```python
from build123d import *

# Parameters (mm, degrees)
SKETCH1_W                      = 600
SKETCH1_H                      = 600
BOSS_EXTRUDE1_DEPTH            = 60
BOSS_EXTRUDE2_START            = 100
SKETCH2_R                      = 20
BOSS_EXTRUDE2_DEPTH            = 100
BOSS_EXTRUDE3_START            = -200
SKETCH2_2_R                    = 20
BOSS_EXTRUDE3_DEPTH            = 100
CUT_EXTRUDE1_REACH             = 677.574
SKETCH2_3_R                    = 20
CUT_EXTRUDE1_DIRECTION_2_REACH = 677.574
FILLET1_R                      = 50


with BuildPart() as part:
    # Sketch1 → Boss-Extrude1 (new body)
    with BuildSketch(Plane(origin=(0, 0, 0), x_dir=(1, 0, 0), z_dir=(0, 1, 0))):
        with Locations((300, 300)):
            Rectangle(SKETCH1_W, SKETCH1_H)
    extrude(amount=BOSS_EXTRUDE1_DEPTH)

    # Sketch2 → Boss-Extrude2 (add)
    with BuildSketch(Plane.XY.offset(-300).offset(BOSS_EXTRUDE2_START)):
        with Locations((0, 60)):
            Circle(SKETCH2_R)
    extrude(amount=BOSS_EXTRUDE2_DEPTH)

    # Sketch2<2> → Boss-Extrude3 (add)
    with BuildSketch(Plane.XY.offset(-300).offset(BOSS_EXTRUDE3_START)):
        with Locations((0, 60)):
            Circle(SKETCH2_2_R)
    extrude(amount=BOSS_EXTRUDE3_DEPTH)

    # Cut-Extrude1: up to this face of the body (flat: up to its plane)
    cut_extrude1_end = Plane(part.part.faces().sort_by_distance((-2.829421211, 62.829421211, -400))[0])
    # Sketch2<3> → Cut-Extrude1 (cut, up to the picked face)
    with BuildSketch(Plane.XY.offset(-300), mode=Mode.PRIVATE) as cut_extrude1_sk1:
        with Locations((0, 60)):
            Circle(SKETCH2_3_R)
    cut_extrude1_tool1 = split(extrude(cut_extrude1_sk1.sketch, amount=-CUT_EXTRUDE1_REACH, mode=Mode.PRIVATE), bisect_by=cut_extrude1_end, keep=Keep.BOTH, mode=Mode.PRIVATE)
    add(cut_extrude1_tool1.solids().sort_by(Axis((0, 60, -300), (0, 0, -1)))[0], mode=Mode.SUBTRACT)

    # Cut-Extrude1 direction 2: up to this face of the body (flat: up to its plane)
    cut_extrude1_direction_2_end = Plane(part.part.faces().sort_by_distance((-2.829421211, 62.829421211, -200))[0])
    # Sketch2<3> → Cut-Extrude1 direction 2 (cut, up to the picked face)
    with BuildSketch(Plane.XY.offset(-300), mode=Mode.PRIVATE) as cut_extrude1_direction_2_sk1:
        with Locations((0, 60)):
            Circle(SKETCH2_3_R)
    cut_extrude1_direction_2_tool1 = split(extrude(cut_extrude1_direction_2_sk1.sketch, amount=CUT_EXTRUDE1_DIRECTION_2_REACH, mode=Mode.PRIVATE), bisect_by=cut_extrude1_direction_2_end, keep=Keep.BOTH, mode=Mode.PRIVATE)
    add(cut_extrude1_direction_2_tool1.solids().sort_by(Axis((0, 60, -300), (0, 0, 1)))[0], mode=Mode.SUBTRACT)

    # Fillet1
    fillet1_edges = [part.edges().sort_by_distance(p)[0] for p in [
        (600, 60, -300),
        (300, 60, -600),
        (600, 30, -600),
        (600, 30, 0),
        (300, 60, 0),
    ]]
    fillet(fillet1_edges, radius=FILLET1_R)


solid = part.part
```
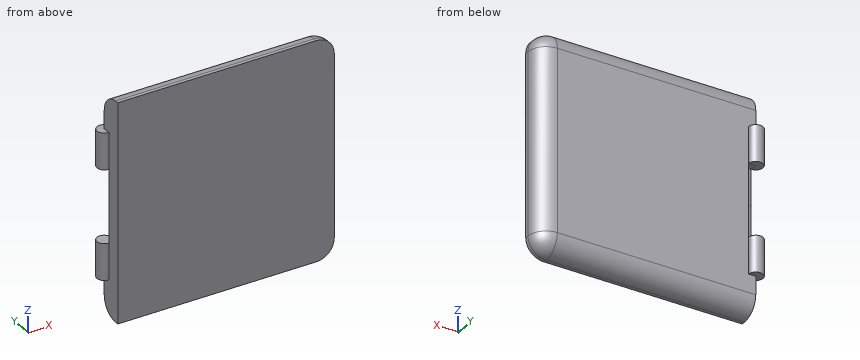
CAD build for the part. Positions are in the model's coordinates, mm. Round coordinates to 2 decimals unless told otherwise and drop trailing zeros. Order: outer loops, then holes, each group sorted by start corner. A loop starts at its lowest first (then second) coordinate and runs counter-clockwise, first axis right, second up. Notation, with made-up numbers: (45.25, 64) -> (98.25, 64) arc R7 ccw to (98.25, 69) -> close; hole circle Ø8 at (57, 6.25). An arc over 180 degrees is marked (long way). One line per question, with ' | ' between items.
Q1. Probe probe 1 along Y at (x, z) = (155, -266.5); probe 2 along Z at (x, y) = (486, 11.5); probe 3 along X at (y, z) = (5, -163.5). List the from-to ranges inside material, lowest first.
Completed:
probe 1: y = 0 to 60 | probe 2: z = -599.98 to -0.02 | probe 3: x = 0 to 600
Q2. Slice it at A-A (x = 405). Write the cut outline in (y, z), then the cut area to 3 significant figures.
Completed:
outline: (0, -600) -> (10, -600) arc R50 ccw to (60, -550) -> (60, -50) arc R50 ccw to (10, 0) -> (0, 0) -> close | area: 34,900 mm^2
Q3. Slice it at B-B (z = -60). Write the cut outline in (x, y).
Completed:
outline: (0, 0) -> (600, 0) -> (600, 10) arc R50 ccw to (550, 60) -> (0, 60) -> close
Q4. Drop flat-ended pins along their axis: pin 1 (2 mm diameter, centred on x = 228.5, z = -110.5, fed in from +Y); pin 2 (4 mm diameter, centred on x = 180, y = 25.5, fed in from +Z); pin 3 (22 mm diameter, centred on x = 6, y = 48.5, fed in from -Z); pin 4 (5 mm diameter, centred on y = 71, z = -96, fed in from +X). Give the stop position or say it passes through.
Completed:
pin 1: stops at y = 60 | pin 2: stops at z = -1.86 | pin 3: stops at z = -591.76 | pin 4: passes through
Q5. Slice it at C-C (y = 21.5). Write the cut outline in (x, z), then the cut area to 3 significant figures.
Completed:
outline: (0, -598.66) -> (550, -598.66) arc R48.66 ccw to (598.66, -550) -> (598.66, -50) arc R48.66 ccw to (550, -1.34) -> (0, -1.34) -> close | area: 357,000 mm^2
